from build123d import *

# Parameters (mm, degrees)
SKETCH1_R           = 7.9
SKETCH1_R_2         = 2.6
BOSS_EXTRUDE1_DEPTH = 4.8
FILLET1_R           = 0.3


with BuildPart() as part:
    # Sketch1 → Boss-Extrude1 (new body)
    with BuildSketch(Plane.XY):
        Circle(SKETCH1_R)
        Circle(SKETCH1_R_2, mode=Mode.SUBTRACT)
    extrude(amount=BOSS_EXTRUDE1_DEPTH)

    # Sketch2 → Cut-Revolve1 (revolve, cut)
    with BuildSketch(Plane(origin=(0, 0, 0), x_dir=(0, 0, -1), z_dir=(1, 0, 0)), mode=Mode.PRIVATE) as cut_revolve1_sk:
        Polygon((-5.02377309, 7.3), (-4.492956226, 7.3), (-4.492956226, 6.942652627), (-4.330576131, 6.780272532), (-4.330576131, 6.378958324), (-4.524078417, 6.185456038), (-4.242386553, 5.903764175), (-4.519629847, 5.626520881), (-4.519629847, 3.272939667), (-3.81743033, 3.272939667), (-3.81743033, 3.2), (-4.879732163, 3.2), (-4.879732163, 0), (-5.869193326, 0), (-5.869193326, 7.3), align=None)
    cut_revolve1 = revolve(cut_revolve1_sk.sketch.rotate(Axis((0, 0, 4.879732163), (0, 0, 1)), 90), axis=Axis((0, 0, 4.879732163), (0, 0, 1)), mode=Mode.SUBTRACT)

    # Mirror1: Cut-Revolve1 across plane
    add(cut_revolve1.mirror(Plane.XY.offset(2.4)), mode=Mode.SUBTRACT)

    # Fillet1
    fillet1_edges = [part.edges().sort_by_distance(p)[0] for p in [
        (-7.9, 0, 0),
        (-7.9, 0, 4.8),
    ]]
    fillet(fillet1_edges, radius=FILLET1_R)


solid = part.part
Could you check a few things on this model? Use its own coordinates, in mm. A direction names the side the tool comes from. Give positions to 0.01 mm unless a question says otherwise; leave off trailing zeros. Order: outer loops, then holes, each group sorted by start corner. A loop starts at its lowest first (then second) coordinate and runs counter-clockwise, first axis right, second up.
Item 1: If we mould it in two halves opening along Y, with no side actions, what happens to faces 1 (the face through (-2.422, 2.422, 0.28)), 2 (the face through (0, 3, 0)), 3 (the face through (-6.269, -4.807, 2.371))? For each: pulls with the +Y half, pulls with the -Y half, needs draft (parallel to the pull), parting line crosses it, or undercut.
Item 2: I need wall thicknesses on line 1 (Y direction, x = 0, z = 1.2); line 2 (Y direction, x = 1.75, z = 0.2); line 3 (Z direction, x = -4.5, y = -0.5). Which ranges of each line are inside material? Lowest first, please.
Item 3: If we section it at A-A, the plane z = 1.9: Write out the boundary of the cut face in (x, y), plus the area to 3 significant figures.
Item 4: I'm going to push flat-ended pins straight in: pin 1 (1.5 mm diameter, centred on y = 1, z = 0.5, fed in from -X); pin 2 (2 mm diameter, centred on x = -3.5, z = 1.5, fed in from +Y). Where does each tip first touch, or does it pass through?
Item 5: For faces 4 (the face through (-2.422, 2.422, 4.52)), 5 (the face through (-0.338, 2.578, 2.366)), which set-ups out of +Z, -Z, +X, -X, +Y, -Y let a thin tool reach every point of the face, with its end or its side?
Values:
1. face 1: undercut
1. face 2: needs draft
1. face 3: parting line crosses it
2. line 1: y = -7.9 to -2.6, 2.6 to 7.9
2. line 2: y = -7.69 to -7.09, -2.68 to -1.92, 1.92 to 2.68, 7.09 to 7.69
2. line 3: z = 0.28 to 4.52
3. outline: circle Ø15.8 at (0, 0); hole circle Ø5.2 at (0, 0)
3. area: 175 mm2
4. pin 1: stops at x = -7.9
4. pin 2: stops at y = 7.49
5. face 4: +Z
5. face 5: +Z, -Z
